The model under review builds one solid part; all positions refer to its coordinate system, in mm. A direction names the side the tool comes from. Coordinates: 2 decimals unless noted, no trailing zeros. Loops run counter-clockwise (first coordinate to the right, second up) from the corner with the lowest first, then second, coordinate; pieces in that order, holes last. Notation, with made-up numbers: (40, 79.5) - (67, 79.5) arc R25 ccw to (67, 116.5) - close; hole circle Ø6 at (-35, -37). An arc over 180 degrees is marked (long way). Answer in a Markdown table with one row per item. Add a question column.
(1) Mouldability with a two-part tool opening along X and no side actions: class faces 3 (the flat face through (-115, 0, 2)), 4 (the flat face through (1, 34, -99.05)), 5 (the flat face through (130.95, 34, 2)) as +X half, -X half, draft (parallel to the pull), parting line (faces both ways), or undercut.
(2) We need section B-B on y = 28. Write out the cut boundary in (x, z).
(3) We need section C-C on z = -20.5. Write out the cut boundary in (x, y).
(4) Machinability: for faces 1 (the flat face through (-1, 34, 99.05)), 2 (the flat face through (-2, 34, 131.25)), which of the approach directions +Z, -Z, +X, -X, +Y, -Y give a long, thin tool a straight path to every point of the face, cutting with its end or side? Answer none if there is none.
(5) We need section A-A on x = 50.5. Write out the cut boundary in (y, z), plus the area to 3 significant figures.
(6) For line 1 along X through (y, z) = (63.5, 27); line 2 along Z through (x, y) = (50, 43.5), list the stretches that pass through material, from the lowest coordinate up.
Autodesk Inventor part; units mm, degrees
ref_plane "YZ Plane" through (0, 0, 0) normal (1, 0, 0) x (0, 1, 0)
ref_plane "XZ Plane" through (0, 0, 0) normal (0, 1, 0) x (-1, 0, 0)
ref_plane "XY Plane" through (0, 0, 0) normal (0, 0, 1) x (1, 0, 0)
sketch "Esboço1" plane through (0, 0, 0) normal (0, 1, 0) x (-1, 0, 0)
  line L0 (130.95, 131.25) -> (-130.95, 131.25)
  line L1 (-130.95, 131.25) -> (-130.95, -131.25)
  line L2 (-130.95, -131.25) -> (130.95, -131.25)
  line L3 (130.95, -131.25) -> (130.95, 131.25)
  line L4 (130.95, 131.25) -> (-130.95, -131.25) construction
  line L5 (-130.95, 131.25) -> (130.95, -131.25) construction
  line L6 (130.95, 99.05) -> (-130.95, 99.05)
  line L7 (-130.95, -99.05) -> (130.95, -99.05)
  line L8 (-99.75, 131.25) -> (-99.75, -131.25)
  line L9 (99.75, -131.25) -> (99.75, 131.25)
  point P0 (0, 0)
  point P1 (99.75, -99.05)
  point P2 (99.75, 99.05)
  point P3 (-99.75, 99.05)
  point P4 (-99.75, -99.05)
  dimension "d0" = 261.9
  dimension "d1" = 262.5
  dimension "d2" = 32.2
  dimension "d3" = 32.2
  dimension "d4" = 31.2
  dimension "d5" = 31.2
extrude "Extrusão1" add sketch "Esboço1" along normal blind 69.3
extrude "Extrusão2" cut sketch "Esboço1" along normal blind 69.3 contours L9 L7 L8 L6
properties part number "NinhoColmeia"
Outcome:
| question | item | result |
|---|---|---|
| 1 | face 3 | draft |
| 1 | face 4 | undercut |
| 1 | face 5 | +X half |
| 2 | outline | (-130.95, -131.25) - (130.95, -131.25) - (130.95, 131.25) - (-130.95, 131.25) - close; hole (-99.75, -99.05) - (99.75, -99.05) - (99.75, 99.05) - (-99.75, 99.05) - close |
| 3 | outline | (-130.95, 0) - (-99.75, 0) - (-99.75, 69.3) - (-130.95, 69.3) - close; (99.75, 0) - (130.95, 0) - (130.95, 69.3) - (99.75, 69.3) - close |
| 4 | face 1 | +Y, -Y |
| 4 | face 2 | +Z, +X, -X, +Y, -Y |
| 5 | outline | (0, -131.25) - (69.3, -131.25) - (69.3, -99.05) - (0, -99.05) - close; (0, 99.05) - (69.3, 99.05) - (69.3, 131.25) - (0, 131.25) - close |
| 5 | area | 4,460 mm² |
| 6 | line 1 | -130.95 to -99.75, 99.75 to 130.95 |
| 6 | line 2 | -131.25 to -99.05, 99.05 to 131.25 |
